Design review of the part built by this model. Coordinates are the model's own, in mm. Face numbers are marked on the shaded views. A direction names the side the tool comes from. Give positions to 0.01 mm unless a question says otherwise; leave off trailing zeros. Loops run counter-clockwise (first coordinate to the right, second up) from the corner with the lowest first, then second, coordinate; pieces in that order, holes last. Notation, with made-up numbers: (-15, 17.5) -> (40, 17.5) arc R25 cw to (40, 46.5) -> close; hole circle Ø8 at (-38.75, 35.25). An arc over 180 degrees is marked (long way). Use a Markdown table: item, result. Add a question column.
1. Add section B-B (y = -1). State the section outline as (x, z) points.
2. Add section A-A (z = 0). State the section outline as (x, y) points, and give its area (3 significant figures).
3. Add section C-C (x = 0). State the section outline as (y, z) points.
4. For pin 1 Ø8.5 at (x, z) = (0.5, 1.5) entering from -Y; pin 2 Ø2 at (y, z) = (2.5, -6.5) entering from -X; pin 3 Ø2.5 at (x, z) = (0, 0) entering from +Y, all flat-tipped, find the tip position at first contact; note any pin that passes through.
5. Add section D-D (y = 0.5). State the section outline as (x, z) points, and give its area (3 significant figures).
6. To check wall thickness, follow line 1 (Y direction, x = -7.5, z = 0.5); line 2 (X direction, y = 6.4, z = 0); line 3 (Z direction, x = 6.5, y = 3.5). State the ranges of each line that lie inside material, in increasing order.
7. Draft analysis for pull direction Z (two halves, no side actions). For the marked faces 1, 2 and 3, state which applies: pulls with the +Z half, pulls with the -Z half, needs draft (parallel to the pull), parting line crosses it, or undercut.
8. For the marked faces 4 and 5, list the 3-axis set-ups (+Z, -Z, +X, -X, +Y, -Y) from which the entire face can be reached by the end or side of a thin tool; tool diameter is ignored.
```python
from build123d import *
from OCP.BRepFilletAPI import BRepFilletAPI_MakeChamfer

# Parameters (mm, degrees)
SKETCH1_R           = 8.5
BOSS_EXTRUDE1_DEPTH = 7.8
SKETCH2_R           = 8.5
SKETCH2_R_2         = 7.8
SKETCH2_R_3         = 1.5
CUT_EXTRUDE1_DEPTH  = 1.5
SKETCH3_R           = 0.5
BOSS_EXTRUDE2_DEPTH = 2
CHAMFER1_SIZE       = 0.5
CHAMFER1_SIZE2      = 0.1
FILLET1_R           = 1
SKETCH4_R           = 7.8
CUT_EXTRUDE2_DEPTH  = 1.3
SKETCH5_R           = 8.5
SKETCH5_R_2         = 7.8
BOSS_EXTRUDE3_DEPTH = 0.2
FILLET2_R           = 1


with BuildPart() as part:
    # Sketch1 → Boss-Extrude1 (new body)
    with BuildSketch(Plane(origin=(0, 0, 0), x_dir=(1, 0, 0), z_dir=(0, 1, 0))):
        with Locations(Location((0, 0, 0), (0, 0, 270))):
            Circle(SKETCH1_R)
    extrude(amount=BOSS_EXTRUDE1_DEPTH)

    # Sketch2 → Cut-Extrude1 (cut)
    with BuildSketch(Plane(origin=(0, 7.8, 0), x_dir=(1, 0, 0), z_dir=(0, 1, 0))):
        with Locations(Location((0, 0, 0), (0, 0, 270))):
            Circle(SKETCH2_R)
        with Locations(Location((0, 0, 0), (0, 0, 270))):
            Circle(SKETCH2_R_2, mode=Mode.SUBTRACT)
        with Locations(Location((0, 0, 0), (0, 0, 270))):
            Circle(SKETCH2_R_3)
    extrude(amount=-CUT_EXTRUDE1_DEPTH, mode=Mode.SUBTRACT)

    # Sketch3 → Boss-Extrude2 (add)
    with BuildSketch(Plane.XZ):
        with Locations(Location((-5, 5, 0), (0, 0, 90))):
            Circle(SKETCH3_R)
        with Locations(Location((5, -5, 0), (0, 0, 90))):
            Circle(SKETCH3_R)
    extrude(amount=BOSS_EXTRUDE2_DEPTH)

    # Chamfer1: one chamfer whose edges measure the first distance from different faces: ONE call of the kernel's chamfer builder (chamfer() names one face for all edges)
    chamfer1_edges_1 = [part.edges().sort_by_distance(p)[0] for p in [
        (-5, -2, 4.5),
    ]]
    chamfer1_side_1 = [part.faces().sort_by_distance(p)[0] for p in [
        (-5, -1, 4.5),
    ]]
    chamfer1_edges_2 = [part.edges().sort_by_distance(p)[0] for p in [
        (5, -2, -5.5),
    ]]
    chamfer1_side_2 = [part.faces().sort_by_distance(p)[0] for p in [
        (5, -1, -5.5),
    ]]
    chamfer1 = BRepFilletAPI_MakeChamfer(part.part.solid().wrapped)
    for e in chamfer1_edges_1:
        chamfer1.Add(CHAMFER1_SIZE, CHAMFER1_SIZE2, e.wrapped, chamfer1_side_1[0].wrapped)  # the first distance lies on this face
    for e in chamfer1_edges_2:
        chamfer1.Add(CHAMFER1_SIZE, CHAMFER1_SIZE2, e.wrapped, chamfer1_side_2[0].wrapped)  # the first distance lies on this face
    add(Compound.cast(chamfer1.Shape()), mode=Mode.REPLACE)

    # Fillet1
    fillet1_edges = [part.edges().sort_by_distance(p)[0] for p in [
        (-5, -1.5, 4.5),
        (5, -1.5, -5.5),
    ]]
    fillet(fillet1_edges, radius=FILLET1_R)

    # Sketch4 → Cut-Extrude2 (cut)
    with BuildSketch(Plane(origin=(0, 7.8, 0), x_dir=(1, 0, 0), z_dir=(0, 1, 0))):
        with Locations(Location((0, 0, 0), (0, 0, 270))):
            Circle(SKETCH4_R)
    extrude(amount=-CUT_EXTRUDE2_DEPTH, mode=Mode.SUBTRACT)

    # Sketch5 → Boss-Extrude3 (add)
    with BuildSketch(Plane(origin=(0, 6.3, 0), x_dir=(1, 0, 0), z_dir=(0, 1, 0))):
        with Locations(Location((0, 0, 0), (0, 0, 270))):
            Circle(SKETCH5_R)
        Circle(SKETCH5_R_2, mode=Mode.SUBTRACT)
    extrude(amount=BOSS_EXTRUDE3_DEPTH)

    # Fillet2
    fillet2_edges = [part.edges().sort_by_distance(p)[0] for p in [
        (0, 6.5, -8.5),
    ]]
    fillet(fillet2_edges, radius=FILLET2_R)


solid = part.part
```
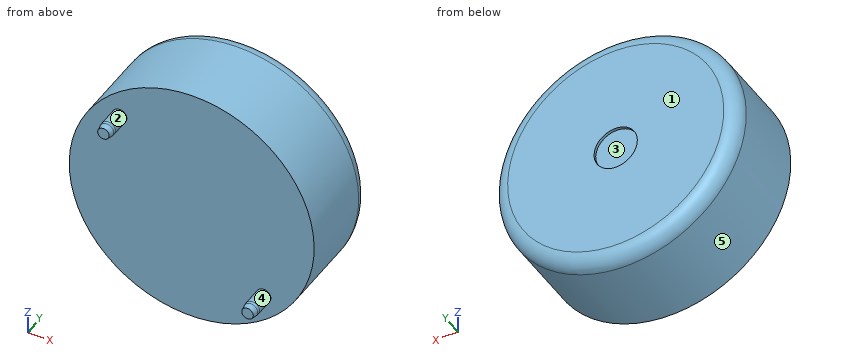
Taken from the geometry:
| question | item | result |
|---|---|---|
| 1 | outline | circle Ø1 at (-5, 5); circle Ø1 at (5, -5) |
| 2 | outline | (-8.5, 0) -> (8.5, 0) -> (8.5, 5.5) arc R1 ccw to (7.5, 6.5) -> (1.5, 6.5) -> (1.5, 6.3) -> (-1.5, 6.3) -> (-1.5, 6.5) -> (-7.5, 6.5) arc R1 ccw to (-8.5, 5.5) -> close |
| 2 | area | 109 mm^2 |
| 3 | outline | (0, -8.5) -> (5.5, -8.5) arc R1 ccw to (6.5, -7.5) -> (6.5, -1.5) -> (6.3, -1.5) -> (6.3, 1.5) -> (6.5, 1.5) -> (6.5, 7.5) arc R1 ccw to (5.5, 8.5) -> (0, 8.5) -> close |
| 4 | pin 1 | stops at y = 0 |
| 4 | pin 2 | stops at x = -6.48 |
| 4 | pin 3 | stops at y = 6.3 |
| 5 | outline | circle Ø17 at (0, 0) |
| 5 | area | 227 mm^2 |
| 6 | line 1 | y = 0 to 6.5 |
| 6 | line 2 | x = -7.94 to -1.5, 1.5 to 7.94 |
| 6 | line 3 | z = -5.48 to 5.48 |
| 7 | face 1 | needs draft |
| 7 | face 2 | parting line crosses it |
| 7 | face 3 | undercut |
| 8 | face 4 | -Y |
| 8 | face 5 | +Y, -Y |
